The listing builds one solid part. Answer for the finished solid, in the listing's coordinates (mm). A direction names the side the tool comes from. Coordinates: 2 decimals unless noted, no trailing zeros. Write each loop counter-clockwise with the first axis right and the second up, starting at its lowest first coordinate (ties: lowest second). Pieces come first, ordered by that corner, then holes.
from build123d import *

# Parameters (mm, degrees)
ESQUISSE1_W             = 34.7
ESQUISSE1_H             = 30.7
BOSS_EXTRU_1_DEPTH      = 8
ESQUISSE2_R             = 3.5
ESQUISSE2_R_2           = 1.25
BOSS_EXTRU_2_DEPTH      = 4.5
ESQUISSE3_W             = 8
ESQUISSE3_H             = 30.7
BOSS_EXTRU_3_DEPTH      = 9.4
ESQUISSE4_R             = 1.25
ENL_V_MAT_EXTRU_1_DEPTH = 31.7
ESQUISSE6_R             = 1.25
ENL_V_MAT_EXTRU_2_DEPTH = 9


with BuildPart() as part:
    # Esquisse1 → Boss.-Extru.1 (new body)
    with BuildSketch(Plane.XY):
        with Locations((-17.35, 0)):
            Rectangle(ESQUISSE1_W, ESQUISSE1_H)
    extrude(amount=BOSS_EXTRU_1_DEPTH)

    # Esquisse2 → Boss.-Extru.2 (add, symmetric)
    with BuildSketch(Plane.XY.offset(8)):
        with Locations((-30.3, 6.95)):
            Circle(ESQUISSE2_R)
        with Locations((-30.3, 6.95)):
            Circle(ESQUISSE2_R_2, mode=Mode.SUBTRACT)
        with Locations((-12, -11.35)):
            Circle(ESQUISSE2_R)
        with Locations((-12, -11.35)):
            Circle(ESQUISSE2_R_2, mode=Mode.SUBTRACT)
    extrude(amount=BOSS_EXTRU_2_DEPTH, both=True)

    # Esquisse3 → Boss.-Extru.3 (add)
    with BuildSketch(Plane.XY.offset(8)):
        with Locations((-4, 0)):
            Rectangle(ESQUISSE3_W, ESQUISSE3_H)
    extrude(amount=BOSS_EXTRU_3_DEPTH)

    # Esquisse4 → Enlèv. mat.-Extru.1 (cut, through all)
    with BuildSketch(Plane(origin=(0, 15.35, 0), x_dir=(1, 0, 0), z_dir=(0, 1, 0))):
        with Locations((-4, -14)):
            Circle(ESQUISSE4_R)
        with Locations((-4, -4)):
            Circle(ESQUISSE4_R)
        with Locations((-17, -4)):
            Circle(ESQUISSE4_R)
        with Locations((-30, -4)):
            Circle(ESQUISSE4_R)
    extrude(amount=-ENL_V_MAT_EXTRU_1_DEPTH, mode=Mode.SUBTRACT)

    # Esquisse6 → Enlèv. mat.-Extru.2 (cut, through all)
    with BuildSketch(Plane.XY.offset(8)):
        with Locations((-30.3, 6.95)):
            Circle(ESQUISSE6_R)
        with Locations((-12, -11.35)):
            Circle(ESQUISSE6_R)
    extrude(amount=-ENL_V_MAT_EXTRU_2_DEPTH, mode=Mode.SUBTRACT)


solid = part.part
Q1. Which of the six approach directions +Z, -Z, +X, -X, +Y, -Y give full straight-line access (tool end or side, diameter ignored) to faces 1 (the face through (-4.16, 0.21, 12.76)), 2 (the face through (-12, -13, 12.5)), 3 (the face through (-26.96, 8, 10.22))?
Answers below:
face 1: +Y, -Y
face 2: +Z, -X, +Y, -Y
face 3: +Z
Q2. The part is cut by section A-A, the plane z = 10.75. Write down the section's boundary in (x, y), then the cut area to 3 significant figures.
Answers below:
outline: circle Ø7 at (-30.3, 6.95); circle Ø7 at (-12, -11.35); (-8, -15.35) - (0, -15.35) - (0, 15.35) - (-8, 15.35) - close; hole circle Ø2.5 at (-30.3, 6.95); hole circle Ø2.5 at (-12, -11.35)
area: 313 mm2
Q3. Determine the mould class of faces 4 (the face through (-22, 0, 8)), 5 (the face through (-14, -15.35, 5)), 6 (the face through (-8, 0, 13)), 7 (the face through (0, 0, 9)) for opening direction X: released by +X, released by -X, zero draft, split by the parting line, or undercut.
Answers below:
face 4: undercut
face 5: zero draft
face 6: undercut
face 7: released by +X
Q4. The part is cut by section C-C, the plane z = 14.75. Write down the section's boundary in (x, y).
Answers below:
outline: (-8, -15.35) - (-5, -15.35) - (-5, 15.35) - (-8, 15.35) - close; (-3, -15.35) - (0, -15.35) - (0, 15.35) - (-3, 15.35) - close
Q5. Find the intervals of material crossed by probe 1 along X at (y, z) = (-4.5, 4); probe 2 along Y at (x, z) = (-12, 11.45); probe 3 along X at (y, z) = (-11.35, 4.25), in increasing order.
Answers below:
probe 1: x = -34.7 to -31.25, -28.75 to -18.25, -15.75 to -5.25, -2.75 to 0
probe 2: y = -14.85 to -12.6, -10.1 to -7.85
probe 3: x = -34.7 to -31.22, -28.78 to -18.22, -15.78 to -13.25, -10.75 to -5.22, -2.78 to 0
Q6. The part is cut by section D-D, the plane x = -12. Write down the section's boundary in (y, z), then the cut area to 3 significant figures.
Answers below:
outline: (-15.35, 0) - (-12.6, 0) - (-12.6, 12.5) - (-14.85, 12.5) - (-14.85, 8) - (-15.35, 8) - close; (-10.1, 0) - (15.35, 0) - (15.35, 8) - (-7.85, 8) - (-7.85, 12.5) - (-10.1, 12.5) - close
area: 246 mm2
Q7. Given pin 1 (2 mm diameter, centred on x = -14.5, y = -11, fed in from +Z); pin 2 (7.5 mm diameter, centred on y = -4.5, z = 14.5, fed in from -X); pin 3 (1.5 mm diameter, centred on x = -27.5, z = 12, fed in from +Y), each flat-ended and moving along its own axis, determine where each tip first touches the part or whether it passes through.
Answers below:
pin 1: stops at z = 12.5
pin 2: stops at x = -8
pin 3: stops at y = 9.79
Q8. The part is cut by section B-B, the plane y = -11.35. Write down the section's boundary in (x, z), then the cut area to 3 significant figures.
Answers below:
outline: (-34.7, 0) - (-13.25, 0) - (-13.25, 12.5) - (-15.5, 12.5) - (-15.5, 8) - (-34.7, 8) - close; (-10.75, 0) - (0, 0) - (0, 17.4) - (-8, 17.4) - (-8, 8) - (-8.5, 8) - (-8.5, 12.5) - (-10.75, 12.5) - close; hole circle Ø2.5 at (-30, 4); hole circle Ø2.5 at (-17, 4); hole circle Ø2.5 at (-4, 4); hole circle Ø2.5 at (-4, 14)
area: 333 mm2
